Here's how the part is built. I have some questions about the finished solid (model axes, mm). Face numbers are marked on the shaded views. Coordinates: 2 decimals unless noted, no trailing zeros. Write each loop counter-clockwise with the first axis right and the second up, starting at its lowest first coordinate (ties: lowest second). Pieces come first, ordered by that corner, then holes.
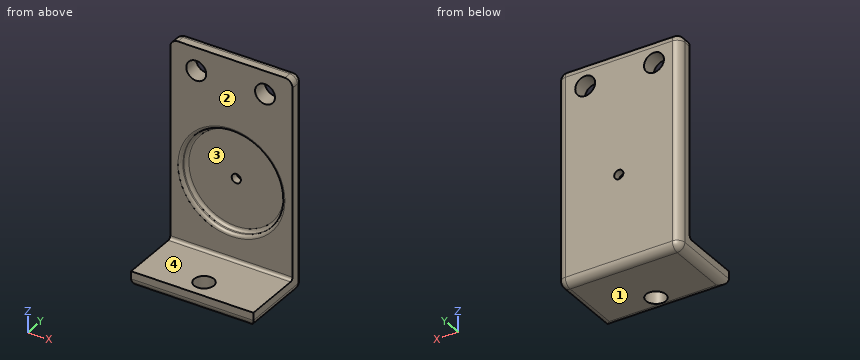
```python
from build123d import *

# Parameters (mm, degrees)
BOSS_EXTRUDE1_DEPTH = 80
SKETCH2_R           = 6.5
CUT_EXTRUDE1_DEPTH  = 167.132477258
SKETCH3_R           = 33
CUT_EXTRUDE2_DEPTH  = 5
FILLET1_R           = 2
SKETCH4_R           = 6.5
CUT_EXTRUDE3_DEPTH  = 158.797338381
FILLET2_R           = 5
FILLET3_R           = 2
SKETCH5_R           = 3
CUT_EXTRUDE4_DEPTH  = 168.406690428


with BuildPart() as part:
    # Sketch1 → Boss-Extrude1 (new body)
    with BuildSketch(Plane(origin=(0, 0, 0), x_dir=(0, 0, -1), z_dir=(1, 0, 0))):
        Polygon((0, 0), (130, 0), (130, -40), (140, -40), (140, 10), (0, 10), align=None)
    extrude(amount=BOSS_EXTRUDE1_DEPTH)

    # Sketch2 → Cut-Extrude1 (cut, through all)
    with BuildSketch(Plane.XZ):
        with Locations(Location((17, -15, 0), (0, 0, 270))):
            Circle(SKETCH2_R)
        with Locations(Location((62, -15, 0), (0, 0, 270))):
            Circle(SKETCH2_R)
    extrude(amount=-CUT_EXTRUDE1_DEPTH, mode=Mode.SUBTRACT)

    # Sketch3 → Cut-Extrude2 (cut)
    with BuildSketch(Plane.XZ):
        with Locations(Location((40, -80, 0), (0, 0, 270))):
            Circle(SKETCH3_R)
    extrude(amount=-CUT_EXTRUDE2_DEPTH, mode=Mode.SUBTRACT)

    # Fillet1
    fillet1_edges = [part.edges().sort_by_distance(p)[0] for p in [
        (40, 5, -47),
        (40, 0, -47),
    ]]
    fillet(fillet1_edges, radius=FILLET1_R)

    # Sketch4 → Cut-Extrude3 (cut, through all)
    with BuildSketch(Plane.XY.offset(-130)):
        with Locations((40, -28)):
            Circle(SKETCH4_R)
    extrude(amount=-CUT_EXTRUDE3_DEPTH, mode=Mode.SUBTRACT)

    # Fillet2
    fillet2_edges = [part.edges().sort_by_distance(p)[0] for p in [
        (40, 10, 0),
        (40, 10, -140),
        (40, -40, -140),
        (80, -15, -140),
        (80, 10, -70),
        (80, 5, 0),
        (0, 10, -70),
        (0, -15, -140),
        (0, 5, 0),
    ]]
    fillet(fillet2_edges, radius=FILLET2_R)

    # Fillet3
    fillet3_edges = [part.edges().sort_by_distance(p)[0] for p in [
        (40, 0, -130),
    ]]
    fillet(fillet3_edges, radius=FILLET3_R)

    # Sketch5 → Cut-Extrude4 (cut, through all)
    with BuildSketch(Plane.XZ.offset(-5)):
        with Locations(Location((40, -80, 0), (0, 0, 270))):
            Circle(SKETCH5_R)
    extrude(amount=-CUT_EXTRUDE4_DEPTH, mode=Mode.SUBTRACT)


solid = part.part
```
1) Imagine slicing it at D-D on y = -10. Please give me the cut outline in (x, z).
Values follow:
outline: (0, -135) arc R5 ccw to (5, -140) - (75, -140) arc R5 ccw to (80, -135) - (80, -130) - (0, -130) - close
2) We'd pull the mould along Z, two halves only. Please class the marked faces 1, 2, 3 and 4: pulls with the +Z half, pulls with the -Z half, needs draft (parallel to the pull), parting line crosses it, or undercut.
Values follow:
face 1: pulls with the -Z half
face 2: needs draft
face 3: undercut
face 4: pulls with the +Z half
3) Will these pins go through, and if not, where does the flat tip stop? pin 1 (8 mm diameter, centred on x = 17, z = -15, fed in from +Y); pin 2 (1.5 mm diameter, centred on x = 9, z = -106.5, fed in from -Y); pin 3 (19 mm diameter, centred on x = 25, y = -17, fed in from +Z).
Values follow:
pin 1: passes through
pin 2: stops at y = 0
pin 3: stops at z = -130
4) Imagine slicing it at A-A on y = -28. Please give me the cut outline in (x, z).
Values follow:
outline: (0, -135) arc R5 ccw to (5, -140) - (33.5, -140) - (33.5, -130) - (0, -130) - close; (46.5, -140) - (75, -140) arc R5 ccw to (80, -135) - (80, -130) - (46.5, -130) - close
5) Imagine slicing it at C-C on z = -80. Please give me the cut outline in (x, y).
Values follow:
outline: (0, 0) - (5, 0) arc R2 ccw to (7, 2) - (7, 3) arc R2 cw to (9, 5) - (37, 5) - (37, 10) - (5, 10) arc R5 ccw to (0, 5) - close; (43, 5) - (71, 5) arc R2 cw to (73, 3) - (73, 2) arc R2 ccw to (75, 0) - (80, 0) - (80, 5) arc R5 ccw to (75, 10) - (43, 10) - close
6) I need wall thicknesses on probe 1 along X at (y, z) = (2.75, -15); probe 2 along X at (y, z) = (6.5, -15); probe 3 along X at (y, z) = (2, -79.5). Which ranges of each line are inside material? Lowest first, please.
Values follow:
probe 1: x = 0 to 10.5, 23.5 to 55.5, 68.5 to 80
probe 2: x = 0.23 to 10.5, 23.5 to 55.5, 68.5 to 79.77
probe 3: x = 0 to 7, 73 to 80
7) Imagine slicing it at B-B on z = -15. Please give me the cut outline in (x, y).
Values follow:
outline: (0, 0) - (10.5, 0) - (10.5, 10) - (5, 10) arc R5 ccw to (0, 5) - close; (23.5, 0) - (55.5, 0) - (55.5, 10) - (23.5, 10) - close; (68.5, 0) - (80, 0) - (80, 5) arc R5 ccw to (75, 10) - (68.5, 10) - close
